CAD build for the part. Positions are in the model's coordinates, mm. A direction names the side the tool comes from. Coordinates: 2 decimals unless noted, no trailing zeros. Order: outer loops, then holes, each group sorted by start corner. A loop starts at its lowest first (then second) coordinate and runs counter-clockwise, first axis right, second up. Notation, with made-up numbers: (57.5, 13) - (94.5, 13) arc R38 ccw to (94.5, 51) - close; hole circle Ø6 at (-8, 52). An arc over 180 degrees is marked (long way). Use one line per item in the form item = value.
Autodesk Inventor part; units mm, degrees
ref_plane "YZ Plane" through (0, 0, 0) normal (1, 0, 0) x (0, 1, 0)
ref_plane "XZ Plane" through (0, 0, 0) normal (0, 1, 0) x (-1, 0, 0)
ref_plane "XY Plane" through (0, 0, 0) normal (0, 0, 1) x (1, 0, 0)
sketch "スケッチ1" plane through (0, 0, 0) normal (0, 0, 1) x (1, 0, 0)
  line L0 (0, 0) -> (0, -25)
  line L1 (0, -25) -> (20, -25)
  line L2 (20, -25) -> (40, -80)
  line L3 (40, -80) -> (100, -80)
  line L4 (100, -80) -> (120, -25)
  line L5 (120, -25) -> (140, -25)
  line L6 (140, -25) -> (140, 0)
  line L7 (140, 0) -> (0, 0)
  line L8 (0, -20) -> (140, -20) construction
  line L9 (0, -10) -> (140, -10) construction
  circle A0 centre (10, -10) radius 2.5
  circle A1 centre (130, -10) radius 2.5
  dimension "d14" = 20
  dimension "d15" = 25
  dimension "d16" = 140
  dimension "d17" = 20
  dimension "d18" = 60
  dimension "d19" = 60
  dimension "d20" = 5
  dimension "d21" = 10
  dimension "d22" = 10
  dimension "d23" = 10
extrude "押し出し3" add sketch "スケッチ1" along normal blind 5
sketch "スケッチ3" plane through (0, 0, 5) normal (0, 0, 1) x (1, 0, 0)
  line L0 (0, 0) -> (0, -25)
  line L1 (0, -20) -> (0, -25)
  line L2 (0, -25) -> (20, -25)
  line L3 (0, -25) -> (20, -25)
  line L4 (20, -25) -> (40, -80)
  line L5 (20, -25) -> (40, -80)
  line L6 (40, -80) -> (100, -80)
  line L7 (40, -80) -> (100, -80)
  line L8 (120, -25) -> (140, -25)
  line L9 (100, -80) -> (120, -25)
  line L10 (120, -25) -> (140, -25)
  line L11 (140, -25) -> (140, 0)
  line L12 (140, -25) -> (140, -20)
  line L13 (140, -20) -> (116.8182, -20)
  line L14 (116.8182, -20) -> (96.8182, -75)
  line L15 (96.8182, -75) -> (43.1818, -75)
  line L16 (43.1818, -75) -> (23.1818, -20)
  line L17 (23.1818, -20) -> (0, -20)
  line L18 (100, -80) -> (120, -25)
  line L19 (43.1818, -75) -> (45, -80) construction
  dimension "d26" = 5
  dimension "d28" = 5
  dimension "d29" = 5
extrude "押し出し4" add sketch "スケッチ3" along normal blind 20
sketch "スケッチ4" plane through (116.8182, -20, 5) normal (0, 1, 0) x (1, 0, 0)
  line L0 (23.1818, 5) -> (23.1818, -20) construction
  line L1 (23.1818, -10) -> (-116.4286, -10) construction
  line L2 (23.1818, -20) -> (0, -20) construction
  circle A0 centre (13.1818, -10) radius 2.5
  circle A1 centre (-106.8182, -10) radius 2.5
  line L3 (-116.8182, 0) -> (-116.8182, -20) construction
  point P0 (-116.8182, 5)
  dimension "d32" = 10
  dimension "d33" = 10
  dimension "d34" = 5
  dimension "d35" = 10
extrude "押し出し5" cut sketch "スケッチ4" against normal blind 20
fillet "フィレット1" radius 5 3 edges at (33.1818, -47.5, 5) (70, -75, 5) (106.8182, -47.5, 5)
fillet "フィレット1" radius 5 6 edges at (20, -25, 12.5) (120, -25, 12.5) (43.1818, -75, 15) (96.8182, -75, 15) (40, -80, 12.5) (100, -80, 12.5)
properties part number "エンコーダガード2"
Item 1: Drop flat-ended pins along their axis: pin 1 (10 mm diameter, centred on x = 19.5, z = 11, fed in from +Y); pin 2 (4 mm diameter, centred on x = 130, z = 15, fed in from -Y); pin 3 (3 mm diameter, centred on x = 107, y = -11, fed in from +Z); pin 4 (12 mm diameter, centred on y = -64, z = 3, fed in from -X). Give the stop position or say it passes through.
Derived:
pin_1 = -20
pin_2 = through
pin_3 = 5
pin_4 = 32
Item 2: Cut at A-A, the plane x = 10. Write the cut outline in (y, z), plus the area to 3 significant figures.
Derived:
outline = (-25, 0) - (-12.5, 0) - (-12.5, 5) - (-20, 5) - (-20, 12.5) - (-25, 12.5) - close; (-25, 17.5) - (-20, 17.5) - (-20, 25) - (-25, 25) - close; (-7.5, 0) - (0, 0) - (0, 5) - (-7.5, 5) - close
area = 175 mm²
Item 3: Two-plate mould, pull along X, no slides. Class faces 3 (the face through (99.4, -79.07, 12.32)), 4 (the face through (43.78, -74.07, 17.6)), 5 (the face through (70, -77, 25)): +X half, -X half, draft (parallel to the pull), parting line (faces both ways), or undercut.
Derived:
face_3 = +X half
face_4 = undercut
face_5 = draft
Item 4: 3-axis set-ups, long thin cutter, end or side, ignore diameter. For faces 1 (the face through (69, -27, 5)), 2 (the face through (71, 0, 2)): which of +Z, -Z, +X, -X, +Y, -Y reach the whole face in a straight line?
Derived:
face_1 = +Z, +Y
face_2 = +Z, -Z, +X, -X, +Y
Item 5: Cut at C-C, the plane z = 15. Write the cut outline in (x, y).
Derived:
outline = (0, -25) - (7.5, -25) - (7.5, -20) - (0, -20) - close; (12.5, -25) - (16.5, -25) arc R5 cw to (21.2, -28.29) - (38.8, -76.71) arc R5 ccw to (43.5, -80) - (96.5, -80) arc R5 ccw to (101.2, -76.71) - (118.8, -28.29) arc R5 cw to (123.5, -25) - (127.5, -25) - (127.5, -20) - (116.82, -20) - (98.02, -71.71) arc R5 cw to (93.32, -75) - (46.68, -75) arc R5 cw to (41.98, -71.71) - (23.18, -20) - (12.5, -20) - close; (132.5, -25) - (140, -25) - (140, -20) - (132.5, -20) - close
Item 6: Drill centre lines: line 1 (Z direction, x = 10, y = -23.55); line 2 (Y direction, x = 10, z = 3.55); line 3 (Y direction, x = 63.5, z = 24). Where is each one in solid material? Low to high. Write a range as [from, to].
Derived:
line_1 = [0, 12.5], [17.5, 25]
line_2 = [-25, -12.5], [-7.5, 0]
line_3 = [-80, -75]
Item 7: Cut at D-D, the plane z = 3.25. Write the cut outline in (x, y).
Derived:
outline = (0, -25) - (16.5, -25) arc R5 cw to (21.2, -28.29) - (38.8, -76.71) arc R5 ccw to (43.5, -80) - (96.5, -80) arc R5 ccw to (101.2, -76.71) - (118.8, -28.29) arc R5 cw to (123.5, -25) - (140, -25) - (140, 0) - (0, 0) - close; hole circle Ø5 at (10, -10); hole circle Ø5 at (130, -10)
Item 8: Cut at B-B, the plane y = -10. Write the cut outline in (x, z).
Derived:
outline = (0, 0) - (7.5, 0) - (7.5, 5) - (0, 5) - close; (12.5, 0) - (127.5, 0) - (127.5, 5) - (12.5, 5) - close; (132.5, 0) - (140, 0) - (140, 5) - (132.5, 5) - close
